Answer from the drawing. Dimensions are ordinates in mm from the lowest x, y and z of the part. A direction names the side the tool comes from. Round coordinates to 2 decimals unless told otherwise and drop trailing zeros. Write each loop counter-clockwise with the first axis right and the second up, starting at its lowest first coordinate (ties: lowest second). Pieces come first, ordered by that corner, then holes. Notation, with made-up numbers: (-37.75, -0.75) - (-33.75, -0.75) arc R8 cw to (-33.75, 3.25) - close; hole circle Ø9 at (4, 27.5). An arc over 180 degrees is marked (long way). One line per item, written item: value. Start each with the question number.
(1) Flat-ended cylindrical pins translate along their axes: pin 1 Ø2 at (y, z) = (6, 5.5) entering from +X; pin 2 Ø1.5 at (x, y) = (2, 9.5) entering from -Z; pin 3 Ø1.8 at (x, z) = (4, 3.5) entering from -Y. Find the tip coordinate at first contact, or state that the pin passes through.
(2) A cutting plane is placed at B-B, the plane x = 5.5. Determine the outline of the cut face in (y, z).
(3) For the marked faces 1 and 2, determine the directions among +Z, -Z, +X, -X, +Y, -Y from which every point of the face is accessible in a straight line to the end or side of a thin tool.
(4) A cutting plane is placed at C-C, the plane y = 1.25. Determine the outline of the cut face in (x, z).
(5) Find the intervals of material crossed by L1, parallel to Y at x = 5.25, z = 5.15; L2, parallel to Z at x = 3.1, y = 2.75; L3, parallel to X at y = 4, z = 2.7, in increasing order.
(6) A cutting plane is placed at A-A, the plane y = 10.5. Determine the outline of the cut face in (x, z).
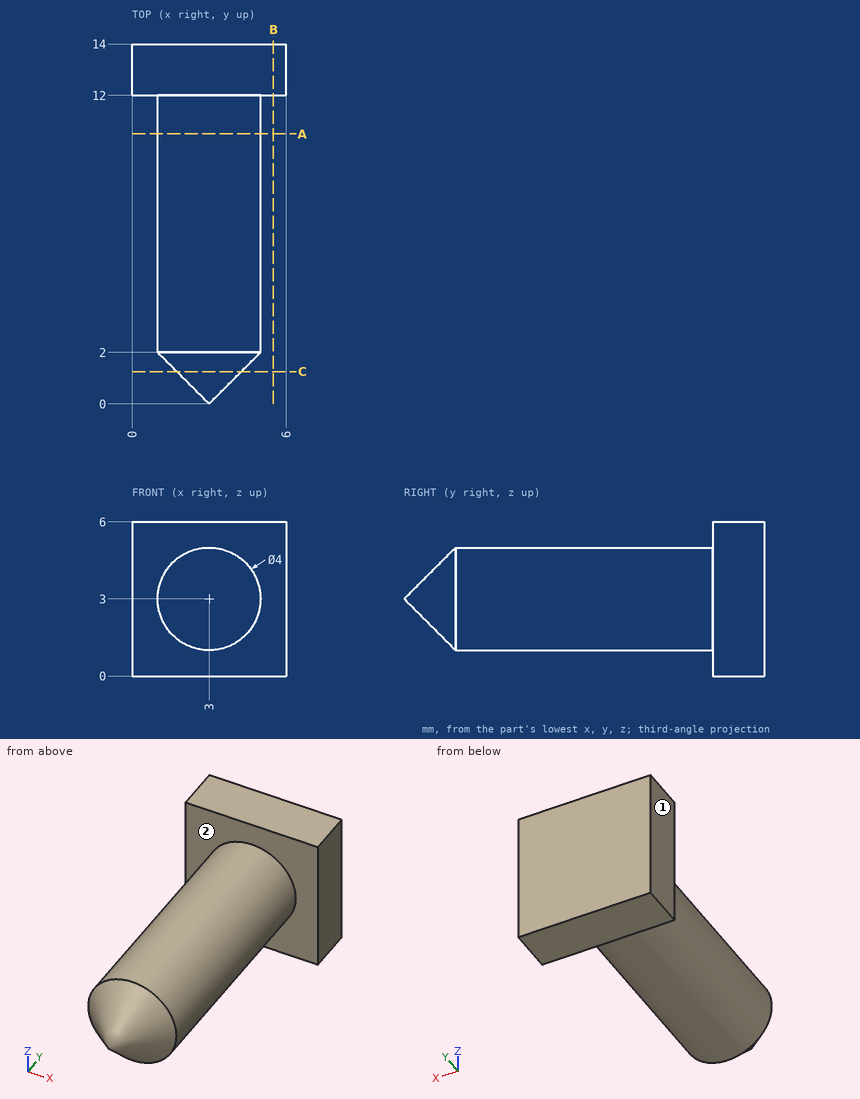
Here are the results:
1. pin 1: x = 4.32
1. pin 2: z = 1.02
1. pin 3: y = 0.22
2. outline: (12, 0) - (14, 0) - (14, 6) - (12, 6) - close
3. face 1: +Z, -Z, -X, +Y, -Y
3. face 2: -Y
4. outline: circle Ø2.5 at (3, 3)
5. L1: 12 to 14
5. L2: 1 to 5
5. L3: 1.02 to 4.98
6. outline: circle Ø4 at (3, 3)
